from build123d import *

# Parameters (mm, degrees)
F0_W     = 650
F0_H     = 5
F1_DEPTH = 320


with BuildPart() as f1:
    # F0 (on Front) → F1 (new body)
    with BuildSketch(Plane.XZ):
        Rectangle(F0_W, F0_H)
        Polygon((325, 2.5), (325, -2.5), (330, -2.5), (330, 27.5), (325, 27.5), align=None)
        Polygon((-330, -2.5), (-325, -2.5), (-325, 2.5), (-325, 62.5), (-330, 62.5), align=None)
    extrude(amount=F1_DEPTH)


solid = f1.part
Read the model definition and answer for the solid it produces. Units are mm, in the model's axes. A direction names the side the tool comes from. Coordinates: 2 decimals unless noted, no trailing zeros. Order: outer loops, then holes, each group sorted by start corner. A loop starts at its lowest first (then second) coordinate and runs counter-clockwise, first axis right, second up. Notation, with made-up numbers: (86, -13.75) -> (100, -13.75) arc R26 ccw to (100, 23.25) -> close; hole circle Ø10 at (-14, 9). An arc over 180 degrees is marked (long way). Answer as a JSON object with one key per item and string values.
1) A cutting plane is placed at C-C, the plane x = -141.5. Determine the outline of the cut face in (y, z).
Model answer:
{"outline": "(-320, -2.5) -> (0, -2.5) -> (0, 2.5) -> (-320, 2.5) -> close"}
2) A cutting plane is placed at B-B, the plane y = -113.5. Determine the outline of the cut face in (x, z).
Model answer:
{"outline": "(-330, -2.5) -> (330, -2.5) -> (330, 27.5) -> (325, 27.5) -> (325, 2.5) -> (-325, 2.5) -> (-325, 62.5) -> (-330, 62.5) -> close"}
3) A tool of negligible diameter and unlimited length cuts with its end or side. For faces 1 (the face through (325, -158, 15)), 2 (the face through (-5, -158, -2.5)), from which of +Z, -Z, +X, -X, +Y, -Y can it reach the whole face along a straight path? Write none if from no direction.
Model answer:
{"face 1": "+Z, +Y, -Y", "face 2": "-Z, +X, -X, +Y, -Y"}
4) The mould has two halves that part along X. Classify faces 3 (the face through (-330, -158, 30)), 4 (the face through (-325, -158, 32)), 5 (the face through (330, -158, 12)), 6 (the face through (-2, 0, -1)): released by +X, released by -X, zero draft, split by the parting line, or undercut.
Model answer:
{"face 3": "released by -X", "face 4": "undercut", "face 5": "released by +X", "face 6": "zero draft"}
5) Consider line 1 along X through (y, z) = (-207.5, 20); line 2 along Z through (x, y) = (207.5, -14); line 3 along X through (y, z) = (-97.5, 50). Determine where each line is inside the solid, lowest interval first. Write a range as from..to.
Model answer:
{"line 1": "x = -330..-325, 325..330", "line 2": "z = -2.5..2.5", "line 3": "x = -330..-325"}
6) Each of these flat-tipped pins is pushed along its axis until it touches: pin 1 (10 mm diameter, centred on x = -67, y = -93, fed in from +Z); pin 2 (10 mm diameter, centred on y = -44, z = 48.5, fed in from +X); pin 3 (1.5 mm diameter, centred on x = 328.5, y = -109.5, fed in from +Z). Where does it stop, or does it pass through?
Model answer:
{"pin 1": "stops at z = 2.5", "pin 2": "stops at x = -325", "pin 3": "stops at z = 27.5"}
7) A cutting plane is placed at D-D, the plane z = 46. Determine the outline of the cut face in (x, y).
Model answer:
{"outline": "(-330, -320) -> (-325, -320) -> (-325, 0) -> (-330, 0) -> close"}
8) A cutting plane is placed at A-A, the plane z = 17.5. Determine the outline of the cut face in (x, y).
Model answer:
{"outline": "(-330, -320) -> (-325, -320) -> (-325, 0) -> (-330, 0) -> close; (325, -320) -> (330, -320) -> (330, 0) -> (325, 0) -> close"}
